Verification items for the finished model (mm, model axes). Face numbers are marked on the shaded views. Round coordinates to 2 decimals unless told otherwise and drop trailing zeros. Order: outer loops, then holes, each group sorted by start corner. A loop starts at its lowest first (then second) coordinate and runs counter-clockwise, first axis right, second up. Notation, with made-up numbers: M 45,20 L 99,20 A17 cw 99,30 Z; hole C 81.5,84 d9. An arc over 180 degrees is marked long. Use CSV: the item, a comma, the result in double quotes. Start each with the question number.
Q1. Gauge pin test, flat ends, axial feed: pin 1 Ø1 at (x, z) = (-4.5, 7) entering from +Y; pin 2 Ø3 at (y, z) = (-2.5, 2.5) entering from +X. Record the tip position at first contact, or that the pin passes through.
Q2. Mould release check, pull along Y, two halves, no side actions. Record for the marked faces 1, 2 and 3: +Y half, -Y half, draft (parallel to the pull), parting line (faces both ways), or undercut.
Q3. Sectioned sample at A-A (z = 4.5). Enter the section's corners in (x, y).
Q4. Scan lines: line 1 (Y direction, x = 0, z = 7); line 2 (Y direction, x = 2.75, z = 1); line 3 (X direction, y = -10, z = 7.25). Record each from-to range of solid material in increasing order.
```python
from build123d import *

# Parameters (mm, degrees)
SKETCH1_R           = 6
BOSS_EXTRUDE1_DEPTH = 12
SKETCH2_OUTSIDE_W   = 111.456
SKETCH2_OUTSIDE_H   = 108.034
SKETCH2_OUTSIDE_R   = 11.251897502
CUT_EXTRUDE1_DEPTH  = 21.986591899
CUT_EXTRUDE1_DRAFT  = -60
SKETCH3_OUTSIDE_W   = 111.456
SKETCH3_OUTSIDE_H   = 108.034
SKETCH3_OUTSIDE_R   = 11.25
CUT_EXTRUDE3_DEPTH  = 21.986591899
CUT_EXTRUDE3_DRAFT  = -60


with BuildPart() as part:
    # Sketch1 → Boss-Extrude1 (new body)
    with BuildSketch(Plane.XY):
        Polygon((6.552777772, 11.227858989), (-6.447222228, 11.28880151), (-13, 0.060942521), (-6.552777772, -11.227858989), (6.447222228, -11.28880151), (13, -0.060942521), align=None)
        Circle(SKETCH1_R, mode=Mode.SUBTRACT)
    extrude(amount=BOSS_EXTRUDE1_DEPTH)


with BuildPart() as cut_extrude1_tool:
    # Sketch2 outside → Cut-Extrude1 (with draft: the straight prism first)
    with BuildSketch(Plane(origin=(0, 0, 0), x_dir=(-1, 0, 0), z_dir=(0, 0, -1))):
        Rectangle(SKETCH2_OUTSIDE_W, SKETCH2_OUTSIDE_H)
        Circle(SKETCH2_OUTSIDE_R, mode=Mode.SUBTRACT)
    extrude(amount=-CUT_EXTRUDE1_DEPTH)
    # Cut-Extrude1: the draft: its side faces are tilted about the plane it starts from
    cut_extrude1_sides = [cut_extrude1_tool.faces().sort_by_distance(p)[0] for p in [
        (0, -54.017, 10.993295949),
        (-55.728, 0, 10.993295949),
        (0, 54.017, 10.993295949),
        (55.728, 0, 10.993295949),
        (11.251897502, 0, 10.993295949),
    ]]
    draft(cut_extrude1_sides, Plane(origin=(0, 0, 0), x_dir=(-1, 0, 0), z_dir=(0, 0, -1)), CUT_EXTRUDE1_DRAFT)


with BuildPart() as part_1:
    add(part.part)

    # Cut-Extrude1: cut by cut_extrude1_tool
    add(cut_extrude1_tool.part, mode=Mode.SUBTRACT)


with BuildPart() as cut_extrude3_tool:
    # Sketch3 outside → Cut-Extrude3 (with draft: the straight prism first)
    with BuildSketch(Plane.XY.offset(12)):
        Rectangle(SKETCH3_OUTSIDE_W, SKETCH3_OUTSIDE_H)
        Circle(SKETCH3_OUTSIDE_R, mode=Mode.SUBTRACT)
    extrude(amount=-CUT_EXTRUDE3_DEPTH)
    # Cut-Extrude3: the draft: its side faces are tilted about the plane it starts from
    cut_extrude3_sides = [cut_extrude3_tool.faces().sort_by_distance(p)[0] for p in [
        (0, -54.017, 1.006704051),
        (55.728, 0, 1.006704051),
        (0, 54.017, 1.006704051),
        (-55.728, 0, 1.006704051),
        (-11.25, 0, 1.006704051),
    ]]
    draft(cut_extrude3_sides, Plane.XY.offset(12), CUT_EXTRUDE3_DRAFT)


with BuildPart() as part_2:
    add(part_1.part)

    # Cut-Extrude3: cut by cut_extrude3_tool
    add(cut_extrude3_tool.part, mode=Mode.SUBTRACT)


solid = part_2.part
```
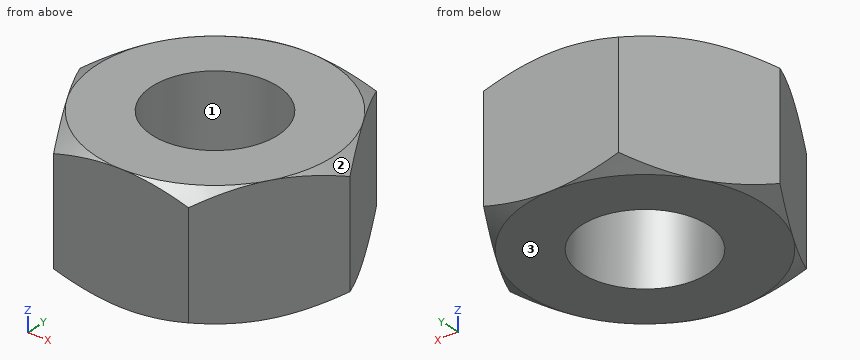
Verdict:
1,pin 1,"stops at y = 11.28"
1,pin 2,"stops at x = 12.45"
2,face 1,"undercut"
2,face 2,"parting line"
2,face 3,"draft"
3,outline,"M -13,0.06 L -6.55,-11.23 L 6.45,-11.29 L 13,-0.06 L 6.55,11.23 L -6.45,11.29 Z; hole C 0,0 d12"
4,line 1,"y = -11.26 to -6, 6 to 11.26"
4,line 2,"y = -11.27 to -5.33, 5.33 to 11.25"
4,line 3,"x = -7.25 to 7.2"
